Could you check a few things on this model? Use its own coordinates, in mm. A direction names the side the tool comes from. Give positions to 0.01 mm unless a question says otherwise; leave off trailing zeros. Write each loop counter-clockwise with the first axis right and the second up, starting at its lowest first coordinate (ties: lowest second). Pieces come first, ordered by that corner, then holes. Notation, with made-up numbers: (-38, 71) -> (-24, 71) arc R31 ccw to (-24, 106) -> close; hole circle Ø7 at (43, 52). An arc over 180 degrees is marked (long way). One line per question, with ' | ' between items.
Autodesk Inventor part; units mm, degrees
ref_plane "YZ Plane" through (0, 0, 0) normal (1, 0, 0) x (0, 1, 0)
ref_plane "XZ Plane" through (0, 0, 0) normal (0, 1, 0) x (-1, 0, 0)
ref_plane "XY Plane" through (0, 0, 0) normal (0, 0, 1) x (1, 0, 0)
sketch "Sketch1" plane through (0, 0, 0) normal (0, 1, 0) x (-1, 0, 0)
  line L0 (12.7, 12.7) -> (12.7, -12.7)
  line L1 (12.7, -12.7) -> (-12.7, -12.7)
  line L2 (-12.7, -12.7) -> (-12.7, 12.7)
  line L3 (-12.7, 12.7) -> (12.7, 12.7)
  line L4 (12.7, 12.7) -> (-12.7, -12.7) construction
  line L5 (12.7, -12.7) -> (-12.7, 12.7) construction
  line L6 (11.1125, 11.1125) -> (11.1125, -11.1125)
  line L7 (11.1125, -11.1125) -> (-11.1125, -11.1125)
  line L8 (-11.1125, -11.1125) -> (-11.1125, 11.1125)
  line L9 (-11.1125, 11.1125) -> (11.1125, 11.1125)
  line L10 (11.1125, 11.1125) -> (-11.1125, -11.1125) construction
  line L11 (11.1125, -11.1125) -> (-11.1125, 11.1125) construction
  point P0 (0, 0)
  dimension "d0" = 25.4
  dimension "d1" = 25.4
  dimension "d2" = 1.5875
  dimension "d3" = 1.5875
extrude "Extrusion1" add sketch "Sketch1" along normal blind 660.4
sketch "Sketch2" plane through (12.7, 0, 12.7) normal (1, 0, 0) x (0, 0, -1)
  line L0 (12.7, 0) -> (12.7, 38.1)
  circle A0 centre (12.7, 38.1) radius 4.7625
  line L1 (3.9688, 38.1) -> (8.3344, 45.6615)
  line L2 (8.3344, 45.6615) -> (17.0656, 45.6615)
  line L3 (17.0656, 45.6615) -> (21.4313, 38.1)
  line L4 (21.4313, 38.1) -> (17.0656, 30.5385)
  line L5 (17.0656, 30.5385) -> (8.3344, 30.5385)
  line L6 (8.3344, 30.5385) -> (3.9688, 38.1)
  dimension "d6" = 38.1
  dimension "d7" = 9.525
  dimension "d8" = 8.7312
extrude "Extrusion2" cut sketch "Sketch2" against normal blind 46.6 contours A0
sketch "Sketch3" plane through (12.7, 0, 12.7) normal (1, 0, 0) x (0, 0, -1)
  line L0 (12.7, 0) -> (12.7, 177.8)
  line L1 (0, 0) -> (0, 660.4)
  line L2 (0, 177.8) -> (180.4268, 177.8)
  line L3 (180.4268, 177.8) -> (180.4268, 742.2297)
  line L4 (180.4268, 742.2297) -> (0, 742.2297)
  line L5 (0, 742.2297) -> (0, 177.8)
  dimension "d11" = 177.8
extrude "Extrusion3" cut sketch "Sketch3" against normal blind 354.85
sketch "Sketch4" plane through (12.7, 0, 12.7) normal (1, 0, 0) x (0, 0, -1)
  point P0 (12.7, 0)
sketch "Sketch5" plane through (-12.7, 0, 12.7) normal (0, 0, 1) x (1, 0, 0)
  line L0 (0, 177.8) -> (25.4, 177.8)
  line L1 (12.7, 177.8) -> (12.7, 165.1)
  circle A0 centre (12.7, 165.1) radius 2.6289
  point P0 (12.7, 0)
  dimension "d14" = 12.7
  dimension "d15" = 5.2578
extrude "Extrusion4" cut sketch "Sketch5" against normal blind 86.1
sketch "Sketch6" plane through (12.7, 0, 12.7) normal (1, 0, 0) x (0, 0, -1)
  circle A0 centre (12.7, 38.1) radius 4.7625
  circle A1 centre (12.7, 38.1) radius 6.35
  point P0 (12.7, 0)
  dimension "d18" = 12.7
extrude "Extrusion5" cut sketch "Sketch6" against normal blind 44.35
properties part number "Tube Finger" material "Aluminum 6061"
Q1. Imagine slicing it at D-D on y = 38.1. Please give me the cut outline in (x, z).
Answer below:
outline: (-12.7, -12.7) -> (12.7, -12.7) -> (12.7, -6.35) -> (11.11, -6.35) -> (11.11, -11.11) -> (-11.11, -11.11) -> (-11.11, -6.35) -> (-12.7, -6.35) -> close; (-12.7, 6.35) -> (-11.11, 6.35) -> (-11.11, 11.11) -> (11.11, 11.11) -> (11.11, 6.35) -> (12.7, 6.35) -> (12.7, 12.7) -> (-12.7, 12.7) -> close
Q2. Imagine slicing it at C-C on z = 0. Please give me the cut outline in (x, y).
Answer below:
outline: (-12.7, 0) -> (-11.11, 0) -> (-11.11, 31.75) -> (-12.7, 31.75) -> close; (-12.7, 44.45) -> (-11.11, 44.45) -> (-11.11, 177.8) -> (-12.7, 177.8) -> close; (11.11, 0) -> (12.7, 0) -> (12.7, 31.75) -> (11.11, 31.75) -> close; (11.11, 44.45) -> (12.7, 44.45) -> (12.7, 177.8) -> (11.11, 177.8) -> close
Q3. Imagine slicing it at B-B on x = 0. Please give me the cut outline in (y, z), and give its area (3 significant figures).
Answer below:
outline: (0, -12.7) -> (162.47, -12.7) -> (162.47, -11.11) -> (0, -11.11) -> close; (0, 11.11) -> (162.47, 11.11) -> (162.47, 12.7) -> (0, 12.7) -> close; (167.73, -12.7) -> (177.8, -12.7) -> (177.8, -11.11) -> (167.73, -11.11) -> close; (167.73, 11.11) -> (177.8, 11.11) -> (177.8, 12.7) -> (167.73, 12.7) -> close | area: 548 mm^2
Q4. If we mould it in two halves opening along Y, with no side actions, what happens to faces 1 (the cylindrical face through (-11.9, 31.9, 1.38)), 2 (the flat face through (0, 88, 11.112)), 3 (the flat face through (11.3, 0, 0.1)), 4 (the cylindrical face through (1.213, 162.768, -11.895))? For each: +Y half, -Y half, draft (parallel to the pull), parting line (faces both ways), or undercut.
Answer below:
face 1: undercut | face 2: draft | face 3: -Y half | face 4: undercut
Q5. On a 3-axis mill with a long thin cutter (end or side, diameter ignored), from which of +Z, -Z, +X, -X, +Y, -Y can I reach the whole of each face in a straight line? I mean faces 5 (the flat face through (-11.112, 88, 0)), 6 (the flat face through (12.7, 88, 0)). Say none if no direction works.
Answer below:
face 5: +Y, -Y | face 6: +Z, -Z, +X, +Y, -Y
Q6. Imagine slicing it at A-A on x = 9. Please give me the cut outline in (y, z).
Answer below:
outline: (0, -12.7) -> (177.8, -12.7) -> (177.8, -11.11) -> (0, -11.11) -> close; (0, 11.11) -> (177.8, 11.11) -> (177.8, 12.7) -> (0, 12.7) -> close
Q7. If I drill on line 1 along X through (y, z) = (141.5, 5); line 2 along X through (y, z) = (165.1, 12.2), over which ranges is the centre line in solid material (lowest first)?
Answer below:
line 1: x = -12.7 to -11.11, 11.11 to 12.7 | line 2: x = -12.7 to -2.63, 2.63 to 12.7
